from build123d import *

# Parameters (mm, degrees)
SKETCH1_W                    = 500
SKETCH1_H                    = 500
BOSS_EXTRUDE1_DEPTH          = 3.175
SKETCH2_W                    = 50
SKETCH2_H                    = 6.35
CUT_EXTRUDE1_DEPTH           = 354.610410622
LPATTERN1_COUNT              = 5
LPATTERN1_PITCH              = 100
SKETCH3_R                    = 5
CUT_EXTRUDE2_DEPTH           = 354.610410622
CIRPATTERN1_COUNT            = 4
CIRPATTERN1_COPY_1_SKETCH_W  = 50
CIRPATTERN1_COPY_1_SKETCH_H  = 6.35
CIRPATTERN1_COPY_1_DEPTH     = 354.610410622
CIRPATTERN1_COPY_2_SKETCH_W  = 50
CIRPATTERN1_COPY_2_SKETCH_H  = 6.35
CIRPATTERN1_COPY_2_DEPTH     = 354.610410622
CIRPATTERN1_COPY_3_SKETCH_W  = 50
CIRPATTERN1_COPY_3_SKETCH_H  = 6.35
CIRPATTERN1_COPY_3_DEPTH     = 354.610410622
CIRPATTERN1_COPY_4_SKETCH_W  = 50
CIRPATTERN1_COPY_4_SKETCH_H  = 6.35
CIRPATTERN1_COPY_4_DEPTH     = 354.610410622
CIRPATTERN1_COPY_5_SKETCH_W  = 50
CIRPATTERN1_COPY_5_SKETCH_H  = 6.35
CIRPATTERN1_COPY_5_DEPTH     = 354.610410622
CIRPATTERN1_COPY_6_SKETCH_W  = 50
CIRPATTERN1_COPY_6_SKETCH_H  = 6.35
CIRPATTERN1_COPY_6_DEPTH     = 354.610410622
CIRPATTERN1_COPY_7_SKETCH_W  = 50
CIRPATTERN1_COPY_7_SKETCH_H  = 6.35
CIRPATTERN1_COPY_7_DEPTH     = 354.610410622
CIRPATTERN1_COPY_8_SKETCH_W  = 50
CIRPATTERN1_COPY_8_SKETCH_H  = 6.35
CIRPATTERN1_COPY_8_DEPTH     = 354.610410622
CIRPATTERN1_COPY_9_SKETCH_W  = 50
CIRPATTERN1_COPY_9_SKETCH_H  = 6.35
CIRPATTERN1_COPY_9_DEPTH     = 354.610410622
CIRPATTERN1_COPY_10_SKETCH_W = 50
CIRPATTERN1_COPY_10_SKETCH_H = 6.35
CIRPATTERN1_COPY_10_DEPTH    = 354.610410622
CIRPATTERN1_COPY_11_SKETCH_W = 50
CIRPATTERN1_COPY_11_SKETCH_H = 6.35
CIRPATTERN1_COPY_11_DEPTH    = 354.610410622
CIRPATTERN1_COPY_12_SKETCH_W = 50
CIRPATTERN1_COPY_12_SKETCH_H = 6.35
CIRPATTERN1_COPY_12_DEPTH    = 354.610410622
SKETCH5_W                    = 6.85
SKETCH5_H                    = 10.5
CUT_EXTRUDE3_DEPTH           = 354.610410622


with BuildPart() as part:
    # Sketch1 → Boss-Extrude1 (new, symmetric)
    with BuildSketch(Plane(origin=(0, 0, 0), x_dir=(1, 0, 0), z_dir=(0, 1, 0))):
        Rectangle(SKETCH1_W, SKETCH1_H)
    extrude(amount=BOSS_EXTRUDE1_DEPTH, both=True)

    # Sketch2 → Cut-Extrude1 (cut, through all)
    with BuildSketch(Plane(origin=(0, 3.175, 0), x_dir=(1, 0, 0), z_dir=(0, 1, 0))):
        with Locations((-225, 246.825)):
            Rectangle(SKETCH2_W, SKETCH2_H)
    cut_extrude1 = extrude(amount=-CUT_EXTRUDE1_DEPTH, mode=Mode.SUBTRACT)

    # LPattern1: Cut-Extrude1 ×5
    with Locations(*[(i * LPATTERN1_PITCH, 0, 0) for i in range(1, LPATTERN1_COUNT)]):
        add(cut_extrude1, mode=Mode.SUBTRACT)

    # Sketch3 → Cut-Extrude2 (cut, through all)
    with BuildSketch(Plane(origin=(0, 3.175, 0), x_dir=(1, 0, 0), z_dir=(0, 1, 0))):
        with Locations(Location((0, 0, 0), (0, 0, 270))):
            Circle(SKETCH3_R)
    extrude(amount=-CUT_EXTRUDE2_DEPTH, mode=Mode.SUBTRACT)

    # CirPattern1: Cut-Extrude1 ×4 about axis
    cirpattern1_axis = Axis((0, 0, 0), (0, 1, 0))
    for i in range(1, CIRPATTERN1_COUNT):
        add(cut_extrude1.rotate(cirpattern1_axis, i * 360 / CIRPATTERN1_COUNT), mode=Mode.SUBTRACT)

    # CirPattern1 copy 1 sketch → CirPattern1 copy 1 (cut, through all)
    with BuildSketch(Plane(origin=(0, 3.175, -100), x_dir=(0, 0, -1), z_dir=(0, 1, 0))):
        with Locations((-225, 246.825)):
            Rectangle(CIRPATTERN1_COPY_1_SKETCH_W, CIRPATTERN1_COPY_1_SKETCH_H)
    extrude(amount=-CIRPATTERN1_COPY_1_DEPTH, mode=Mode.SUBTRACT)

    # CirPattern1 copy 2 sketch → CirPattern1 copy 2 (cut, through all)
    with BuildSketch(Plane(origin=(-100, 3.175, 0), x_dir=(-1, 0, 0), z_dir=(0, 1, 0))):
        with Locations((-225, 246.825)):
            Rectangle(CIRPATTERN1_COPY_2_SKETCH_W, CIRPATTERN1_COPY_2_SKETCH_H)
    extrude(amount=-CIRPATTERN1_COPY_2_DEPTH, mode=Mode.SUBTRACT)

    # CirPattern1 copy 3 sketch → CirPattern1 copy 3 (cut, through all)
    with BuildSketch(Plane(origin=(0, 3.175, 100), x_dir=(0, 0, 1), z_dir=(0, 1, 0))):
        with Locations((-225, 246.825)):
            Rectangle(CIRPATTERN1_COPY_3_SKETCH_W, CIRPATTERN1_COPY_3_SKETCH_H)
    extrude(amount=-CIRPATTERN1_COPY_3_DEPTH, mode=Mode.SUBTRACT)

    # CirPattern1 copy 4 sketch → CirPattern1 copy 4 (cut, through all)
    with BuildSketch(Plane(origin=(0, 3.175, -200), x_dir=(0, 0, -1), z_dir=(0, 1, 0))):
        with Locations((-225, 246.825)):
            Rectangle(CIRPATTERN1_COPY_4_SKETCH_W, CIRPATTERN1_COPY_4_SKETCH_H)
    extrude(amount=-CIRPATTERN1_COPY_4_DEPTH, mode=Mode.SUBTRACT)

    # CirPattern1 copy 5 sketch → CirPattern1 copy 5 (cut, through all)
    with BuildSketch(Plane(origin=(-200, 3.175, 0), x_dir=(-1, 0, 0), z_dir=(0, 1, 0))):
        with Locations((-225, 246.825)):
            Rectangle(CIRPATTERN1_COPY_5_SKETCH_W, CIRPATTERN1_COPY_5_SKETCH_H)
    extrude(amount=-CIRPATTERN1_COPY_5_DEPTH, mode=Mode.SUBTRACT)

    # CirPattern1 copy 6 sketch → CirPattern1 copy 6 (cut, through all)
    with BuildSketch(Plane(origin=(0, 3.175, 200), x_dir=(0, 0, 1), z_dir=(0, 1, 0))):
        with Locations((-225, 246.825)):
            Rectangle(CIRPATTERN1_COPY_6_SKETCH_W, CIRPATTERN1_COPY_6_SKETCH_H)
    extrude(amount=-CIRPATTERN1_COPY_6_DEPTH, mode=Mode.SUBTRACT)

    # CirPattern1 copy 7 sketch → CirPattern1 copy 7 (cut, through all)
    with BuildSketch(Plane(origin=(0, 3.175, -300), x_dir=(0, 0, -1), z_dir=(0, 1, 0))):
        with Locations((-225, 246.825)):
            Rectangle(CIRPATTERN1_COPY_7_SKETCH_W, CIRPATTERN1_COPY_7_SKETCH_H)
    extrude(amount=-CIRPATTERN1_COPY_7_DEPTH, mode=Mode.SUBTRACT)

    # CirPattern1 copy 8 sketch → CirPattern1 copy 8 (cut, through all)
    with BuildSketch(Plane(origin=(-300, 3.175, 0), x_dir=(-1, 0, 0), z_dir=(0, 1, 0))):
        with Locations((-225, 246.825)):
            Rectangle(CIRPATTERN1_COPY_8_SKETCH_W, CIRPATTERN1_COPY_8_SKETCH_H)
    extrude(amount=-CIRPATTERN1_COPY_8_DEPTH, mode=Mode.SUBTRACT)

    # CirPattern1 copy 9 sketch → CirPattern1 copy 9 (cut, through all)
    with BuildSketch(Plane(origin=(0, 3.175, 300), x_dir=(0, 0, 1), z_dir=(0, 1, 0))):
        with Locations((-225, 246.825)):
            Rectangle(CIRPATTERN1_COPY_9_SKETCH_W, CIRPATTERN1_COPY_9_SKETCH_H)
    extrude(amount=-CIRPATTERN1_COPY_9_DEPTH, mode=Mode.SUBTRACT)

    # CirPattern1 copy 10 sketch → CirPattern1 copy 10 (cut, through all)
    with BuildSketch(Plane(origin=(0, 3.175, -400), x_dir=(0, 0, -1), z_dir=(0, 1, 0))):
        with Locations((-225, 246.825)):
            Rectangle(CIRPATTERN1_COPY_10_SKETCH_W, CIRPATTERN1_COPY_10_SKETCH_H)
    extrude(amount=-CIRPATTERN1_COPY_10_DEPTH, mode=Mode.SUBTRACT)

    # CirPattern1 copy 11 sketch → CirPattern1 copy 11 (cut, through all)
    with BuildSketch(Plane(origin=(-400, 3.175, 0), x_dir=(-1, 0, 0), z_dir=(0, 1, 0))):
        with Locations((-225, 246.825)):
            Rectangle(CIRPATTERN1_COPY_11_SKETCH_W, CIRPATTERN1_COPY_11_SKETCH_H)
    extrude(amount=-CIRPATTERN1_COPY_11_DEPTH, mode=Mode.SUBTRACT)

    # CirPattern1 copy 12 sketch → CirPattern1 copy 12 (cut, through all)
    with BuildSketch(Plane(origin=(0, 3.175, 400), x_dir=(0, 0, 1), z_dir=(0, 1, 0))):
        with Locations((-225, 246.825)):
            Rectangle(CIRPATTERN1_COPY_12_SKETCH_W, CIRPATTERN1_COPY_12_SKETCH_H)
    extrude(amount=-CIRPATTERN1_COPY_12_DEPTH, mode=Mode.SUBTRACT)

    # Sketch5 → Cut-Extrude3 (cut, through all)
    with BuildSketch(Plane(origin=(0, 3.175, 0), x_dir=(1, 0, 0), z_dir=(0, 1, 0))):
        with Locations((-210.225, -201.1)):
            Rectangle(SKETCH5_W, SKETCH5_H)
        with Locations((-210.225, -233.4)):
            Rectangle(SKETCH5_W, SKETCH5_H)
    extrude(amount=-CUT_EXTRUDE3_DEPTH, mode=Mode.SUBTRACT)


solid = part.part
The listing builds one solid part. Answer for the finished solid, in the listing's coordinates (mm). Round coordinates to 2 decimals unless told otherwise and drop trailing zeros. Write item = value, one per line. Start each with the question number.
1) Given pin 1 (1.9 mm diameter, centred on x = -245.5, y = 0.5, fed in from -Z); pin 2 (3 mm diameter, centred on y = 0.5, z = 233.5, fed in from -X); pin 3 (3 mm diameter, centred on y = 0.5, z = 248, fed in from +X), each flat-ended and moving along its own axis, determine where each tip first touches the part or whether it passes through.
2) Straight lines are drawn through the part: L1, parallel to Z at x = 74, y = 2.75; L2, parallel to Z at x = -161, y = 1.75. For each, find the intervals that lie inside material, in ascending order.
3) Section A-A, the plane y = 1 is taken. Count the separate pieces of the cut face and the enclosed holes in it, plus the area to 3 significant figures.
Results list:
q1.pin_1 = -243.65
q1.pin_2 = -243.65
q1.pin_3 = 200
q2.L1 = -243.65 to 250
q2.L2 = -250 to 243.65
q3.separate_pieces = 1
q3.enclosed_holes = 3
q3.area = 243,000 mm^2
